Geometry: see drawing. Coordinates: mm, zero at the bounding-box minimum. Round coordinates to 2 decimals unless told otherwise and drop trailing zeros. Write each loop counter-clockwise with the first axis right and the second up, starting at its lowest first coordinate (ties: lowest second). Pieces come first, ordered by that corner, then holes. Notation, with made-up numbers: M 14.5,-34.5 L 65.5,-34.5 A16 ccw 65.5,-15.5 Z; hole C -0.75,72 d8. An arc over 180 degrees is marked long. Use one line per item in the form item = value. Start each with the question number.
Item 1: Pin query (flat end, axial travel): pin 1 Ø3.5 at (x, y) = (29, 51) entering from +Z; pin 2 Ø1 at (y, z) = (62, 0.5) entering from +X. Return the tip coordinate at first contact, or that it passes through.
Item 2: Ray query, probe 1 along Y at (x, z) = (71, 0.5); probe 2 along Y at (x, z) = (29, 0.7); probe 3 along X at (y, z) = (73.5, 1.85). Return the intervals inside material, ascending.
Item 3: Section query A-A (y = 51). Return loops of the section in (x, z), and give its area (3 significant figures).
Item 4: Section query C-C (z = 0.3). State how many separate pieces and enclosed holes the cut face has, and give its area (3 significant figures).
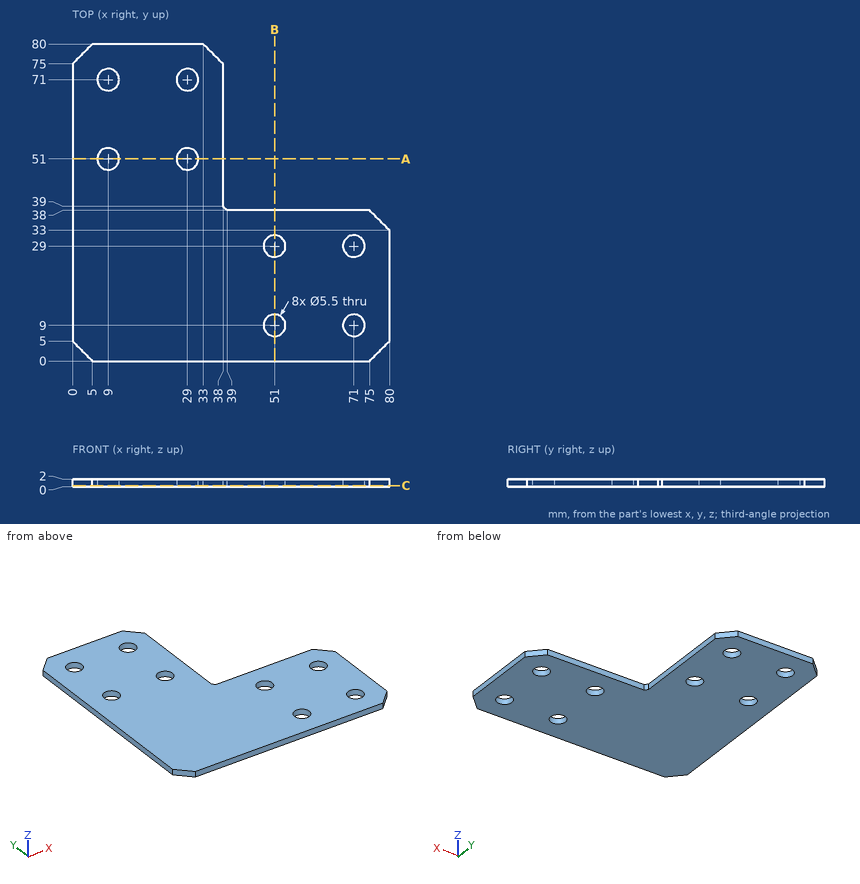
Working result:
q1.pin_1 = through
q1.pin_2 = 38
q2.probe_1 = 0 to 6.25, 11.75 to 26.25, 31.75 to 38
q2.probe_2 = 0 to 48.25, 53.75 to 68.25, 73.75 to 80
q2.probe_3 = 0 to 7.85, 10.15 to 27.85, 30.15 to 38
q3.outline = M 0,0 L 6.25,0 L 6.25,2 L 0,2 Z; M 11.75,0 L 26.25,0 L 26.25,2 L 11.75,2 Z; M 31.75,0 L 38,0 L 38,2 L 31.75,2 Z
q3.area = 54.0 mm²
q4.separate_pieces = 1
q4.enclosed_holes = 8
q4.area = 4,380 mm²
